```python
from build123d import *

# Parameters (mm, degrees)
SKETCH1_R           = 9
SKETCH1_R_2         = 2.35
BOSS_EXTRUDE1_DEPTH = 3
FILLET1_R           = 0.1


with BuildPart() as part:
    # Sketch1 → Boss-Extrude1 (new body)
    with BuildSketch(Plane(origin=(0, 0, 0), x_dir=(1, 0, 0), z_dir=(0, 1, 0))):
        Circle(SKETCH1_R)
        with Locations((4.997281989, -0.164841493)):
            Circle(SKETCH1_R_2, mode=Mode.SUBTRACT)
        Polygon((-2.2, 0.85), (-2.2, -0.85), (-0.85, -0.85), (-0.85, -2.2), (0.85, -2.2), (0.85, -0.85), (2.2, -0.85), (2.2, 0.85), (0.85, 0.85), (0.85, 2.2), (-0.85, 2.2), (-0.85, 0.85), align=None, mode=Mode.SUBTRACT)
    extrude(amount=BOSS_EXTRUDE1_DEPTH)

    # Fillet1
    fillet1_edges = [part.edges().sort_by_distance(p)[0] for p in [
        (-0.85, 1.5, -0.85),
        (-2.2, 1.5, -0.85),
        (-2.2, 1.5, 0.85),
        (-0.85, 1.5, 0.85),
        (-0.85, 1.5, 2.2),
        (0.85, 1.5, 2.2),
        (0.85, 1.5, 0.85),
        (2.2, 1.5, 0.85),
        (2.2, 1.5, -0.85),
        (0.85, 1.5, -0.85),
        (0.85, 1.5, -2.2),
        (-0.85, 1.5, -2.2),
    ]]
    fillet(fillet1_edges, radius=FILLET1_R)


solid = part.part
```
Verification items for the finished model (mm, model axes). A direction names the side the tool comes from. Give positions to 0.01 mm unless a question says otherwise; leave off trailing zeros. Order: outer loops, then holes, each group sorted by start corner. A loop starts at its lowest first (then second) coordinate and runs counter-clockwise, first axis right, second up. Notation, with made-up numbers: M -11,-39.5 L 26,-39.5 A12 ccw 26,-17.5 Z; hole C 77.25,43.25 d9. An arc over 180 degrees is marked long. Return JSON: item names as keys, results as strings. Group by question number.
1) Section check D-D on z = -4.75. Record the cut outline in (x, y), and give its area (3 significant figures).
2) Go/stop test with flat-tipped pins: pin 1 Ø1 at (y, z) = (2.5, 5) entering from -X; pin 2 Ø1.3 at (y, z) = (1.5, -1.5) entering from -X; pin 3 Ø0.6 at (x, y) = (-1.5, 1) entering from -Z. Record where each tip stops, or that it passes through.
3) Section check A-A on x = 0. Record the cut outline in (y, z), and give its area (3 significant figures).
4) Scan lines: line 1 (X direction, y = 2.05, z = -2); line 2 (X direction, y = 2.1, z = 1); line 3 (Z direction, x = -0.5, y = 1.5). Record each from-to range of solid material in increasing order.
5) Section check B-B on z = 1.5. Record the cut outline in (x, y).
6) Access from +Z, -Z, +X, -X, +Y, -Y to the whole of each face (thin tool, end or side, straight path). Record for faces 1 (the face through (-2, 3, 2)), 2 (the face through (1.5, 1.5, 0.85)).
7) Section check C-C on y = 0.4. Record the cut outline in (x, z).
8) Mould release check, pull along X, two halves, no side actions. Record for faces 3 (the face through (1.5, 1.5, -0.85)), 4 (the face through (-1.172, 1.479, -8.923)), 5 (the face through (-2, 0, 2)), 6 (the face through (-1.5, 1.5, 0.85)): pulls with the +X half, pulls with the -X half, needs draft (parallel to the pull), parting line crosses it, or undercut.
Answer block:
{
 "1": {"outline": "M -7.64,0 L 7.64,0 L 7.64,3 L -7.64,3 Z", "area": "45.9 mm^2"},
 "2": {"pin 1": "stops at x = -7.79", "pin 2": "stops at x = -8.96", "pin 3": "stops at z = -8.92"},
 "3": {"outline": "M 0,-9 L 3,-9 L 3,-2.2 L 0,-2.2 Z; M 0,2.2 L 3,2.2 L 3,9 L 0,9 Z", "area": "40.8 mm^2"},
 "4": {"line 1": "x = -8.77 to -0.85, 0.85 to 4.08, 5.91 to 8.77", "line 2": "x = -8.94 to -0.85, 0.85 to 2.8, 7.19 to 8.94", "line 3": "z = -8.99 to -2.2, 2.2 to 8.99"},
 "5": {"outline": "M -8.87,0 L -0.85,0 L -0.85,3 L -8.87,3 Z; M 0.85,0 L 3.06,0 L 3.06,3 L 0.85,3 Z; M 6.93,0 L 8.87,0 L 8.87,3 L 6.93,3 Z"},
 "6": {"face 1": "+Z, -Z, +X, -X, +Y", "face 2": "+Y, -Y"},
 "7": {"outline": "C 0,0 d18; hole M -2.2,-0.75 A0.1 ccw -2.1,-0.85 L -0.95,-0.85 A0.1 cw -0.85,-0.95 L -0.85,-2.1 A0.1 ccw -0.75,-2.2 L 0.75,-2.2 A0.1 ccw 0.85,-2.1 L 0.85,-0.95 A0.1 cw 0.95,-0.85 L 2.1,-0.85 A0.1 ccw 2.2,-0.75 L 2.2,0.75 A0.1 ccw 2.1,0.85 L 0.95,0.85 A0.1 cw 0.85,0.95 L 0.85,2.1 A0.1 ccw 0.75,2.2 L -0.75,2.2 A0.1 ccw -0.85,2.1 L -0.85,0.95 A0.1 cw -0.95,0.85 L -2.1,0.85 A0.1 ccw -2.2,0.75 Z; hole C 5,0.16 d4.7"},
 "8": {"face 3": "undercut", "face 4": "parting line crosses it", "face 5": "needs draft", "face 6": "undercut"}
}
